Model file for the job. Use its own axes, mm. Face numbers are marked on the shaded views. A direction names the side the tool comes from. Give positions to 0.01 mm unless a question says otherwise; leave off trailing zeros. Loops run counter-clockwise (first coordinate to the right, second up) from the corner with the lowest first, then second, coordinate; pieces in that order, holes last. Notation, with made-up numbers: (50, 51) - (78, 51) arc R16 cw to (78, 72) - close; hole circle Ø11 at (44, 80.25). An arc over 180 degrees is marked (long way). Answer as CSV lines item,"result". Start each with the question number.
Item 1: Saw through at B-B on y = 3.25. Give the cut face in (x, z), plus the area to 3 significant figures.
Item 2: Tool access for the marked faces 1, 2 and 3: list every direction of +Z, -Z, +X, -X, +Y, -Y with a clear straight run to the whole face (end or side of a thin tool).
Item 3: Pull direction Y, two halves, no side cores. Call the marked faces 4, 5 and 6: pulls with the +Y half, pulls with the -Y half, needs draft (parallel to the pull), parting line crosses it, or undercut.
Item 4: Pin check, flat tips, straight feed: pin 1 (0.9 mm diameter, centred on x = 0.5, z = -3.5, fed in from -Y); pin 2 (2 mm diameter, centred on y = 1.5, z = -2, fed in from -X). Stop position of each tip, or through.
Item 5: Saw through at A-A on x = 0.75. Give the cut face in (y, z) (3 decimals), plus the area to 3 significant figures.
Item 6: Drill centre lines: L1, parallel to Z at x = 0.75, y = 8.5; L2, parallel to X at y = 3.5, z = -0.5; L3, parallel to Z at x = 0, y = 6. Where is each one in solid material? Low to high. Write a range as from..to.
Item 7: Saw through at C-C on y = 2. Give the cut face in (x, z).
from build123d import *

# Parameters (mm, degrees)
BOSS_EXTRUDE1_DEPTH = 1.5
DRAFT4_ANGLE        = -1
FILLET1_R           = 0.1
SKETCH5_R           = 0.125
CUT_EXTRUDE1_DEPTH  = 2.5


with BuildPart() as part:
    # Sketch1 → Boss-Extrude1 (new body)
    with BuildSketch(Plane(origin=(0, 0, 0), x_dir=(0, 0, -1), z_dir=(1, 0, 0))):
        Polygon((0.9, 1.9), (0.9, 0), (0, 0), (0, 3.674994058), (4, 5.325119328), (4, 7.218922126), (2.71583546, 7.218922126), (2.71583546, 9.5), (6.966077176, 9.5), (6.966077176, 4.107871531), align=None)
    extrude(amount=BOSS_EXTRUDE1_DEPTH)

    # Draft4
    draft4_faces = [part.faces().sort_by_distance(p)[0] for p in [
        (0, 5.526450361, -4.018047871),
        (1.5, 5.526450361, -4.018047871),
    ]]
    draft(draft4_faces, Plane.ZX, DRAFT4_ANGLE)

    # Fillet1
    fillet1_edges = [part.edges().sort_by_distance(p)[0] for p in [
        (1.609478529, 6.272020727, -4),
        (-0.078548782, 4.500056693, -2),
        (-0.109478529, 6.272020727, -4),
        (-0.126006754, 7.218922126, -3.35791773),
        (-0.145914936, 8.359461063, -2.71583546),
        (1.578548782, 4.500056693, -2),
        (0.75, 7.218922126, -4),
        (0.75, 7.218922126, -2.71583546),
        (1.618763141, 6.803935765, -6.966077176),
        (1.645914936, 8.359461063, -2.71583546),
        (1.626006754, 7.218922126, -3.35791773),
        (-0.118763141, 6.803935765, -6.966077176),
    ]]
    fillet(fillet1_edges, radius=FILLET1_R)

    # Sketch5 → Cut-Extrude1 (cut)
    with BuildSketch(Plane(origin=(0, 9.5, 0), x_dir=(1, 0, 0), z_dir=(0, 1, 0))):
        with Locations((0.75, 5.866077176)):
            Circle(SKETCH5_R)
    extrude(amount=-CUT_EXTRUDE1_DEPTH, mode=Mode.SUBTRACT)


solid = part.part
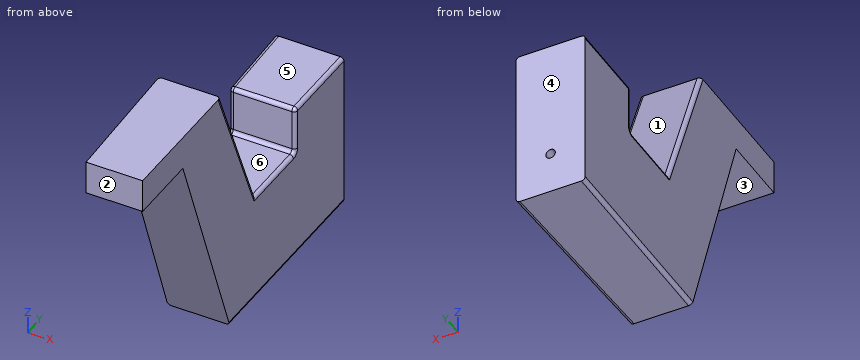
Responses:
1,outline,"(-0.06, -4.61) - (1.56, -4.61) - (1.56, 0) - (-0.06, 0) - close"
1,area,"7.44 mm2"
2,face 1,"+Z, +X, -X"
2,face 2,"+Z, -Z, +X, -X, -Y"
2,face 3,"-Z, +X, -X, -Y"
3,face 4,"pulls with the +Y half"
3,face 5,"needs draft"
3,face 6,"undercut"
4,pin 1,"y = 2.68"
4,pin 2,"x = -0.04"
5,outline,"(0, -0.9) - (1.9, -0.9) - (4.108, -6.966) - (9.5, -6.966) - (9.5, -5.991) - (7, -5.991) - (7, -5.741) - (9.5, -5.741) - (9.5, -2.716) - (7.319, -2.716) arc R0.1 ccw to (7.219, -2.816) - (7.219, -3.9) arc R0.1 cw to (7.119, -4) - (5.325, -4) - (3.675, 0) - (0, 0) - close"
5,area,"30.3 mm2"
6,L1,"-6.97..-5.99, -5.74..-2.72"
6,L2,"-0.06..1.56"
6,L3,"-6.97..-4"
7,outline,"(-0.03, -1.17) - (1.53, -1.17) - (1.53, 0) - (-0.03, 0) - close"
